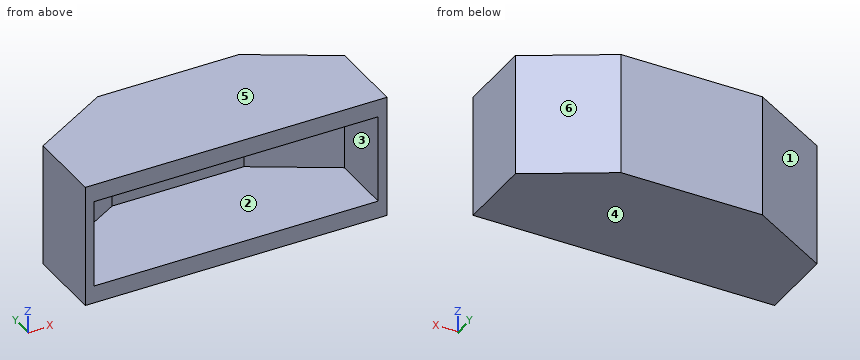
```python
from build123d import *

# Parameters (mm, degrees)
BOSS_EXTRUDE1_DEPTH  = 10
BOSS_EXTRUDE2_DEPTH  = 2
BOSS_EXTRUDE3_DEPTH  = 2
SKETCH4_W            = 32.320508076
SKETCH4_H            = 7
BOSS_EXTRUDE4_DEPTH  = 2
SKETCH5_W            = 32.320508076
SKETCH5_H            = 7
BOSS_EXTRUDE5_DEPTH  = 2
BOSS_EXTRUDE9_DEPTH  = 14
BOSS_EXTRUDE10_DEPTH = 14


with BuildPart() as part:
    # Sketch1 → Boss-Extrude1 (new body)
    with BuildSketch(Plane.XY):
        Polygon((15, 0), (23.660254038, -5), (24.660254038, -3.267949192), (15.535898385, 2), (-0.535898385, 2), (-9.660254038, -3.267949192), (-8.660254038, -5), (0, 0), align=None)
    extrude(amount=BOSS_EXTRUDE1_DEPTH)

    # Sketch2 → Boss-Extrude2 (add)
    with BuildSketch(Plane.XY.offset(10)):
        Polygon((-8.660254038, -5), (23.660254038, -5), (15, 0), (0, 0), align=None)
        Polygon((23.660254038, -5), (24.660254038, -3.267949192), (15.535898385, 2), (-0.535898385, 2), (-9.660254038, -3.267949192), (-8.660254038, -5), (0, 0), (15, 0), align=None)
    extrude(amount=BOSS_EXTRUDE2_DEPTH)

    # Sketch3 → Boss-Extrude3 (add)
    with BuildSketch(Plane(origin=(0, 0, 0), x_dir=(-1, 0, 0), z_dir=(0, 0, -1))):
        Polygon((-24.660254038, -3.267949192), (-15.535898385, 2), (0.535898385, 2), (9.660254038, -3.267949192), (8.660254038, -5), (-23.660254038, -5), align=None)
    extrude(amount=BOSS_EXTRUDE3_DEPTH)

    # Sketch4 → Boss-Extrude4 (add)
    with BuildSketch(Plane.XY.offset(12)):
        with Locations((7.5, -8.5)):
            Rectangle(SKETCH4_W, SKETCH4_H)
    extrude(amount=-BOSS_EXTRUDE4_DEPTH)

    # Sketch5 → Boss-Extrude5 (add)
    with BuildSketch(Plane(origin=(0, 0, -2), x_dir=(-1, 0, 0), z_dir=(0, 0, -1))):
        with Locations((-7.5, -8.5)):
            Rectangle(SKETCH5_W, SKETCH5_H)
    extrude(amount=-BOSS_EXTRUDE5_DEPTH)

    # Sketch8 → Boss-Extrude9 (add)
    with BuildSketch(Plane.XY.offset(12)):
        Polygon((-9.660254038, -3.267949192), (-9.660254038, -12), (-8.660254038, -12), (-8.660254038, -5), align=None)
    extrude(amount=-BOSS_EXTRUDE9_DEPTH)

    # Sketch9 → Boss-Extrude10 (add)
    with BuildSketch(Plane(origin=(0, 0, -2), x_dir=(-1, 0, 0), z_dir=(0, 0, -1))):
        Polygon((-24.660254038, -3.267949192), (-23.660254038, -5), (-23.660254038, -12), (-24.660254038, -12), align=None)
    extrude(amount=-BOSS_EXTRUDE10_DEPTH)


solid = part.part
```
The model under review builds one solid part; all positions refer to its coordinate system, in mm. Face numbers are marked on the shaded views. A direction names the side the tool comes from. Round coordinates to 2 decimals unless told otherwise and drop trailing zeros. Loops run counter-clockwise (first coordinate to the right, second up) from the corner with the lowest first, then second, coordinate; pieces in that order, holes last.
Item 1: Clearance check with flat-ended pins moving along their axes: pin 1 Ø1 at (x, z) = (-1.5, 8.5) entering from -Y; pin 2 Ø5 at (x, z) = (7, 4.5) entering from -Y. State where each tip first meets the part, or that it passes through.
Determined:
pin 1: stops at y = -1.15
pin 2: stops at y = 0
Item 2: For line 1 (Z direction, x = 22, y = -7.75); line 2 (X direction, y = -10.25, z = 0.25); line 3 (Y direction, x = 14.5, z = 8.75), list the stretches that pass through material, from the lowest coordinate up.
Determined:
line 1: z = -2 to 0, 10 to 12
line 2: x = -9.66 to -8.66, 23.66 to 24.66
line 3: y = 0 to 2
Item 3: Take a section at C-C (x = 3). Write out the cut boundary in (y, z), then the cut area to 3 significant figures.
Determined:
outline: (-12, -2) - (2, -2) - (2, 12) - (-12, 12) - (-12, 10) - (0, 10) - (0, 0) - (-12, 0) - close
area: 76.0 mm2
Item 4: Take a section at A-A (y = -5.5). Write out the cut boundary in (x, z), then the cut area to 3 significant figures.
Determined:
outline: (-9.66, -2) - (24.66, -2) - (24.66, 12) - (-9.66, 12) - close; hole (-8.66, 0) - (23.66, 0) - (23.66, 10) - (-8.66, 10) - close
area: 157 mm2
Item 5: Mouldability with a two-part tool opening along Z and no side actions: class the marked faces 3, 4, 5 and 6 as released by +Z, released by -Z, zero draft, split by the parting line, or undercut.
Determined:
face 3: undercut
face 4: released by -Z
face 5: released by +Z
face 6: zero draft
Item 6: Take a section at B-B (z = 8). Write out the cut boundary in (x, y), then the cut area to 3 significant figures.
Determined:
outline: (-9.66, -12) - (-8.66, -12) - (-8.66, -5) - (0, 0) - (15, 0) - (23.66, -5) - (23.66, -12) - (24.66, -12) - (24.66, -3.27) - (15.54, 2) - (-0.54, 2) - (-9.66, -3.27) - close
area: 87.9 mm2
Item 7: For the marked faces 1 and 2, list the 3-axis set-ups (+Z, -Z, +X, -X, +Y, -Y) from which the entire face can be reached by the end or side of a thin tool; tool diameter is ignored.
Determined:
face 1: +Z, -Z, -X, +Y
face 2: -Y
Item 8: Take a section at D-D (x = 17.5). Write out the cut boundary in (y, z), then the cut area to 3 significant figures.
Determined:
outline: (-12, -2) - (0.87, -2) - (0.87, 12) - (-12, 12) - (-12, 10) - (-1.44, 10) - (-1.44, 0) - (-12, 0) - close
area: 74.6 mm2
